Verification items for the finished model (mm, model axes). A direction names the side the tool comes from. Coordinates: 2 decimals unless noted, no trailing zeros. Loops run counter-clockwise (first coordinate to the right, second up) from the corner with the lowest first, then second, coordinate; pieces in that order, holes last. Notation, with made-up numbers: (58, 55.5) -> (63, 55.5) arc R18 ccw to (63, 65.5) -> close; hole circle Ø1 at (0.5, -23). An arc over 180 degrees is marked (long way). Answer as a JSON object with one key per item and string values. Group by question number.
Q1. Scan lines: L1, parallel to Z at x = -8, y = 0.2; L2, parallel to X at y = 0.5, z = -6; L3, parallel to Y at x = -7, z = 0. Record each from-to range of solid material in increasing order.
Q2. Cross-section at A-A on x = 8. Record the boundary of the cut face in (y, z), and give its area (3 significant figures).
Q3. Gauge pin test, flat end, axial feed: pin 1 Ø0.7 at (x, z) = (-2.5, 4.5) entering from +Y. Record the tip position at first contact, or that the pin passes through.
Q4. Set-up check for faces 1 (the flat face through (0, 0, -10)), 2 (the flat face through (-3, 1.5, 0)): record each of +Z, -Z, +X, -X, +Y, -Y from which the full face is reachable in a straight line by a thin tool's end or side.
Q5. Release check for a two-part mould opening along Z. For faces 3 (the cylindrical face through (-9.823, 0.324, 7.043)), 4 (the flat face through (7, 1.5, -9)), 5 (the flat face through (0, 0, 10)) record: released by +Z, released by -Z, zero draft, split by the parting line, or undercut.
Q6. Cross-section at D-D on y = 0.1. Record the boundary of the cut face in (x, z).
Q7. Cross-section at C-C on z = -0.75. Record the boundary of the cut face in (x, y), and give its area (3 significant figures).
Q8. Cross-section at B-B on z = 6. Record the boundary of the cut face in (x, y), and give its area (3 significant figures).
```python
from build123d import *

# Parameters (mm, degrees)
BOSS_EXTRUDE1_DEPTH = 10
SKETCH2_R           = 2.1
CUT_EXTRUDE1_DEPTH  = 16.592786592


with BuildPart() as part:
    # Sketch1 → Boss-Extrude1 (new, symmetric)
    with BuildSketch(Plane.XY):
        Polygon((-11.377389582, 1.5), (-11.122610418, 2.2), (-8.877389582, 2.2), (-8.622610418, 1.5), (-6.377389582, 1.5), (-6.122610418, 2.2), (-3.877389582, 2.2), (-3.622610418, 1.5), (-1.377389582, 1.5), (-1.122610418, 2.2), (1.122610418, 2.2), (1.377389582, 1.5), (3.622610418, 1.5), (3.877389582, 2.2), (6.122610418, 2.2), (6.377389582, 1.5), (8.622610418, 1.5), (8.877389582, 2.2), (11.122610418, 2.2), (11.377389582, 1.5), (11.377389582, -1.5), (-11.377389582, -1.5), align=None)
    extrude(amount=BOSS_EXTRUDE1_DEPTH, both=True)

    # Sketch2 → Cut-Extrude1 (cut, through all)
    with BuildSketch(Plane.XZ.offset(1.5)):
        with Locations(Location((-8, -6, 0), (0, 0, 270))):
            Circle(SKETCH2_R)
        with Locations(Location((8, -6, 0), (0, 0, 287.246374966))):
            Circle(SKETCH2_R)
        with Locations(Location((8, 6, 0), (0, 0, 270))):
            Circle(SKETCH2_R)
        with Locations(Location((-8, 6, 0), (0, 0, 252.753625034))):
            Circle(SKETCH2_R)
    extrude(amount=-CUT_EXTRUDE1_DEPTH, mode=Mode.SUBTRACT)


solid = part.part
```
Computed values:
{
 "1": {"L1": "z = -10 to -8.1, -3.9 to 3.9, 8.1 to 10", "L2": "x = -11.38 to -10.1, -5.9 to 5.9, 10.1 to 11.38", "L3": "y = -1.5 to 1.5"},
 "2": {"outline": "(-1.5, -10) -> (1.5, -10) -> (1.5, -8.1) -> (-1.5, -8.1) -> close; (-1.5, -3.9) -> (1.5, -3.9) -> (1.5, 3.9) -> (-1.5, 3.9) -> close; (-1.5, 8.1) -> (1.5, 8.1) -> (1.5, 10) -> (-1.5, 10) -> close", "area": "34.8 mm²"},
 "3": {"pin 1": "stops at y = 1.5"},
 "4": {"face 1": "-Z, +X, -X, +Y, -Y", "face 2": "+Z, -Z, +Y"},
 "5": {"face 3": "undercut", "face 4": "zero draft", "face 5": "released by +Z"},
 "6": {"outline": "(-11.38, -10) -> (11.38, -10) -> (11.38, 10) -> (-11.38, 10) -> close; hole circle Ø4.2 at (-8, -6); hole circle Ø4.2 at (-8, 6); hole circle Ø4.2 at (8, -6); hole circle Ø4.2 at (8, 6)"},
 "7": {"outline": "(-11.38, -1.5) -> (11.38, -1.5) -> (11.38, 1.5) -> (11.12, 2.2) -> (8.88, 2.2) -> (8.62, 1.5) -> (6.38, 1.5) -> (6.12, 2.2) -> (3.88, 2.2) -> (3.62, 1.5) -> (1.38, 1.5) -> (1.12, 2.2) -> (-1.12, 2.2) -> (-1.38, 1.5) -> (-3.62, 1.5) -> (-3.88, 2.2) -> (-6.12, 2.2) -> (-6.38, 1.5) -> (-8.62, 1.5) -> (-8.88, 2.2) -> (-11.12, 2.2) -> (-11.38, 1.5) -> close", "area": "77.0 mm²"},
 "8": {"outline": "(-11.38, -1.5) -> (-10.1, -1.5) -> (-10.1, 2.2) -> (-11.12, 2.2) -> (-11.38, 1.5) -> close; (-5.9, -1.5) -> (5.9, -1.5) -> (5.9, 2.2) -> (3.88, 2.2) -> (3.62, 1.5) -> (1.38, 1.5) -> (1.12, 2.2) -> (-1.12, 2.2) -> (-1.38, 1.5) -> (-3.62, 1.5) -> (-3.88, 2.2) -> (-5.9, 2.2) -> close; (10.1, -1.5) -> (11.38, -1.5) -> (11.38, 1.5) -> (11.12, 2.2) -> (10.1, 2.2) -> close", "area": "49.4 mm²"}
}
